Autodesk Fusion 360 part; units mm, degrees
sketch "Sketch1" plane through (0, 0, 0) normal (0, 0, 1) x (1, 0, 0) in component "PlugMountSmall"
  line L0 (-13, 25.63) -> (13, 25.63)
  line L1 (13, 25.63) -> (13, 13.63)
  line L2 (13, 13.63) -> (-13, 13.63)
  line L3 (-13, 13.63) -> (-13, 25.63)
  line L4 (0, 25.63) -> (0, 13.63) construction
  line L5 (13, 19.63) -> (-13, 19.63) construction
  line L6 (-0.5, 24.33) -> (0.5, 24.33)
  line L7 (0.5, 24.33) -> (0.5, 14.33)
  line L8 (0.5, 14.33) -> (-0.5, 14.33)
  line L9 (-0.5, 14.33) -> (-0.5, 24.33)
  line L10 (-6, 25.63) -> (-6, 24.53)
  line L11 (-6, 24.53) -> (-5.2, 24.53)
  line L12 (-5.2, 24.53) -> (-5.2, 13.63)
  circle A0 centre (-9, 19.63) radius 1.75
  circle A1 centre (9, 19.63) radius 1.75
  line L13 (5.2, 24.53) -> (5.2, 13.63)
  line L14 (6, 24.53) -> (5.2, 24.53)
  line L15 (6, 25.63) -> (6, 24.53)
  line L16 (-5.2, 24.53) -> (5.2, 24.53)
  dimension "d44_1" = 26
  dimension "d45_1" = 12
  dimension "d46_1" = 10
  dimension "d47_1" = 1.3
  dimension "d48_1" = 1
  dimension "d49_1" = 0.5
  dimension "d50_1" = 3.5
  dimension "d51_1" = 0.8
  dimension "d52_1" = 1.1
  dimension "d53_1" = 7
  dimension "d54_1" = 4
extrude "Extrude1" add sketch "Sketch1" along normal blind 3 contours L2 L12 L13 L16 | L6 L7 L8 L9 in component "PlugMountSmall"
extrude "Extrude2" add sketch "Sketch1" along normal blind 3.3 contours L6 L7 L8 L9 in component "PlugMountSmall"
extrude "Extrude3" add sketch "Sketch1" along normal blind 2 contours L0 L10 L11 L14 L15 L16 in component "PlugMountSmall"
extrude "Extrude4" add sketch "Sketch1" along normal blind 7.7 contours L0 L2 L3 L10 L11 L12 | L0 L1 L2 L13 L14 L15 in component "PlugMountSmall"
component "PlugMountSmall" placed x (1, 0, 0) y (0, 1, 0) z (0, 0, 1) at (0, 0, 0)
Verification items for the finished model (mm, model axes). A direction names the side the tool comes from. Coordinates: 2 decimals unless noted, no trailing zeros. Order: outer loops, then holes, each group sorted by start corner. A loop starts at its lowest first (then second) coordinate and runs counter-clockwise, first axis right, second up. Notation, with made-up numbers: (83, 58) -> (109, 58) arc R19 cw to (109, 89) -> close; hole circle Ø11 at (-14, 69). An arc over 180 degrees is marked (long way). Put each result on its own line as item: value. Start each with the question number.
1) Go/stop test with flat-tipped pins: pin 1 (2 mm diameter, centred on x = -9, y = 19.63, fed in from -Z); pin 2 (0.5 mm diameter, centred on x = 0, y = 17.5, fed in from +Z). Record where each tip stops, or that it passes through.
2) Material ranges on L1, parallel to X at y = 19.5, z = 3.25; L2, parallel to Y at x = -9, z = 4.5; L3, parallel to X at y = 18.5, z = 1, recorded low to high.
3) Cross-section at B-B (y = 19.63). Enter the section's corners in (x, z), plus the area to 3 significant figures.
4) Cross-section at C-C (x = -9). Enter the section's corners in (y, z).
5) Cross-section at D-D (z = 2.25). Enter the section's corners in (x, y).
6) Cross-section at A-A (z = 4.25). Enter the section's corners in (x, y), plus the area to 3 significant figures.
7) Tool access check on faces 1 (the cylindrical face through (-8.19, 21.18, 3.8)), 2 (the flat face through (-6, 25, 5)), 3 (the flat face through (-5.2, 19, 5)). Record the directions out of +Z, -Z, +X, -X, +Y, -Y that give a thin tool (end or side, any length) a straight path to the whole face; none if there is none.
Geometry check:
1. pin 1: passes through
1. pin 2: stops at z = 3.3
2. L1: x = -13 to -10.75, -7.25 to -5.2, -0.5 to 0.5, 5.2 to 7.25, 10.75 to 13
2. L2: y = 13.63 to 17.88, 21.38 to 25.63
2. L3: x = -13 to -10.34, -7.66 to 7.66, 10.34 to 13
3. outline: (-13, 0) -> (-10.75, 0) -> (-10.75, 7.7) -> (-13, 7.7) -> close; (-7.25, 0) -> (7.25, 0) -> (7.25, 7.7) -> (5.2, 7.7) -> (5.2, 3) -> (0.5, 3) -> (0.5, 3.3) -> (-0.5, 3.3) -> (-0.5, 3) -> (-5.2, 3) -> (-5.2, 7.7) -> (-7.25, 7.7) -> close; (10.75, 0) -> (13, 0) -> (13, 7.7) -> (10.75, 7.7) -> close
3. area: 97.7 mm^2
4. outline: (13.63, 0) -> (17.88, 0) -> (17.88, 7.7) -> (13.63, 7.7) -> close; (21.38, 0) -> (25.63, 0) -> (25.63, 7.7) -> (21.38, 7.7) -> close
5. outline: (-13, 13.63) -> (13, 13.63) -> (13, 25.63) -> (6, 25.63) -> (6, 24.53) -> (-6, 24.53) -> (-6, 25.63) -> (-13, 25.63) -> close; hole circle Ø3.5 at (-9, 19.63); hole circle Ø3.5 at (9, 19.63)
6. outline: (-13, 13.63) -> (-5.2, 13.63) -> (-5.2, 24.53) -> (-6, 24.53) -> (-6, 25.63) -> (-13, 25.63) -> close; (5.2, 13.63) -> (13, 13.63) -> (13, 25.63) -> (6, 25.63) -> (6, 24.53) -> (5.2, 24.53) -> close; hole circle Ø3.5 at (-9, 19.63); hole circle Ø3.5 at (9, 19.63)
6. area: 166 mm^2
7. face 1: +Z, -Z
7. face 2: +Z, +Y
7. face 3: +Z, +Y, -Y
